Read the model definition and answer for the solid it produces. Units are mm, in the model's axes. A direction names the side the tool comes from. Give positions to 0.01 mm unless a question says otherwise; leave off trailing zeros. Order: outer loops, then holes, each group sorted by start corner. A loop starts at its lowest first (then second) coordinate and runs counter-clockwise, first axis right, second up. Notation, with made-up numbers: (-1.5, 61.25) -> (21.5, 61.25) arc R27 ccw to (21.5, 85.25) -> close; hole circle Ø11 at (6, 80). An arc over 180 degrees is marked (long way). Answer as CSV lines item,"result". Start each with the question number.
1) Find section A-A (x = 13.5). Determine the outline of the cut face in (y, z), and give its area (3 significant figures).
2) Find section C-C (y = 13). Determine the outline of the cut face in (x, z), and give its area (3 significant figures).
3) Flat-ended cylindrical pins translate along their axes: pin 1 Ø4 at (x, y) = (-1, 3) entering from +Z; pin 2 Ø3.5 at (y, z) = (-7.73, 35.28) entering from +X; pin 3 Ø4 at (y, z) = (14, 2) entering from -X; pin 4 Ø4 at (x, z) = (-11, 1.5) entering from +Y. Find the tip coordinate at first contact, or state that the pin passes through.
4) The mould has two halves that part along Z. Classify faces 1 (the face through (8.42, -20.77, 34.06)), 2 (the face through (20.77, 23.57, 21)), 3 (the face through (2, -19, 19)), 4 (the face through (20.774, 17.714, 11.718)): +Z half, -Z half, draft (parallel to the pull), parting line (faces both ways), or undercut.
5) Straight lines are drawn through the part: L1, parallel to Z at x = -6, y = -11.5; L2, parallel to Z at x = 20.5, y = 17; L3, parallel to X at y = 11, z = 18. For each, find the intervals that lie inside material, in ascending order. Write a range as from..to.
6) For faces 5 (the face through (22.5, -1, 20)), 6 (the face through (19, -2, 19)), 7 (the face through (21, 14, 22.5)), 8 (the face through (-3.5, -21, 33)), determine the directions among +Z, -Z, +X, -X, +Y, -Y from which every point of the face is accessible in a straight line to the end or side of a thin tool.
7) Find section B-B (x = -17). Determine the outline of the cut face in (y, z), and give its area (3 significant figures).
```python
from build123d import *

# Parameters (mm, degrees)
F1_DEPTH  = 44
F2_T      = -3.5
F3_W      = 21.5
F3_H      = 21.5
F4_DEPTH  = 25
F5_W      = 21.5
F5_H      = 21.5
F6_DEPTH  = 25
F7_R      = 5
F10_R     = 1.5
F11_DEPTH = 25
F9_R      = 1.5
F12_DEPTH = 25
F8_R      = 1.5
F13_DEPTH = 25


with BuildPart() as f1:
    # F0 (on Top) → F1 (new body)
    with BuildSketch(Plane.XY):
        Polygon((0, 25), (0, 0), (-25, 0), (-25, -22.5), (0, -22.5), (22.5, -22.5), (22.5, 0), (22.5, 25), align=None)
    extrude(amount=F1_DEPTH)

    # F2
    f2_openings = [f1.faces().sort_by_distance(p)[0] for p in [
        (3.060345, -3.060345, 44),
        (0, 12.5, 22),
        (-12.5, 0, 22),
        (-25, -11.25, 22),
        (11.25, 25, 22),
    ]]
    offset(amount=F2_T, openings=f2_openings)

    # F3 (on face) → F4 (cut)
    with BuildSketch(Plane(origin=(19, 0, 0), x_dir=(0, -1, 0), z_dir=(-1, 0, 0))):
        with Locations((-14.25, 33.25)):
            Rectangle(F3_W, F3_H)
    extrude(amount=-F4_DEPTH, mode=Mode.SUBTRACT)

    # F5 (on face) → F6 (cut)
    with BuildSketch(Plane(origin=(0, -19, 0), x_dir=(-1, 0, 0), z_dir=(0, 1, 0))):
        with Locations((14.25, 33.25)):
            Rectangle(F5_W, F5_H)
    extrude(amount=-F6_DEPTH, mode=Mode.SUBTRACT)

    # F7
    f7_edges = [f1.edges().sort_by_distance(p)[0] for p in [
        (22.5, 1.25, 0),
        (-1.25, -22.5, 0),
        (22.5, -22.5, 22),
        (0, 0, 1.75),
        (-3.5, -20.75, 22.5),
        (0, 25, 1.75),
        (20.75, 25, 22.5),
        (-3.5, -20.75, 44),
        (-25, -20.75, 22.5),
        (-25, 0, 1.75),
        (20.75, 3.5, 22.5),
        (20.75, 3.5, 44),
    ]]
    fillet(f7_edges, radius=F7_R)

    # F10 (on face) → F11 (cut)
    with BuildSketch(Plane.XZ.offset(22.5)):
        with Locations((7.732233047, 35.3934139763)):
            Circle(F10_R)
        with Locations((-16.3934139763, 11.267766953)):
            Circle(F10_R)
    extrude(amount=-F11_DEPTH, mode=Mode.SUBTRACT)

    # F9 (on face) → F12 (cut)
    with BuildSketch(Plane.YZ.offset(22.5)):
        with Locations((-7.732233047, 35.2836836879)):
            Circle(F9_R)
        with Locations((16.2836836879, 11.267766953)):
            Circle(F9_R)
    extrude(amount=-F12_DEPTH, mode=Mode.SUBTRACT)

    # F8 (on face) → F13 (cut)
    with BuildSketch(Plane.XY.offset(3.5)):
        with Locations((-17.0746488054, -8.482233047)):
            Circle(F8_R)
        with Locations((8.482233047, 17.0746488054)):
            Circle(F8_R)
    extrude(amount=-F13_DEPTH, mode=Mode.SUBTRACT)


solid = f1.part
```
Findings below:
1,outline,"(-22.5, 5) arc R5 ccw to (-17.5, 0) -> (25, 0) -> (25, 3.5) -> (-19, 3.5) -> (-19, 44) -> (-22.5, 44) -> close"
1,area,"303 mm²"
2,outline,"(0, 0) -> (17.5, 0) arc R5 ccw to (22.5, 5) -> (22.5, 22.5) -> (19, 22.5) -> (19, 3.5) -> (0, 3.5) -> close"
2,area,"140 mm²"
3,pin 1,"z = 3.5"
3,pin 2,"x = 22.5"
3,pin 3,"x = 0"
3,pin 4,"y = 0"
4,face 1,"undercut"
4,face 2,"+Z half"
4,face 3,"draft"
4,face 4,"undercut"
5,L1,"0..3.5"
5,L2,"1..9.95, 12.59..22.5"
5,L3,"19..22.5"
6,face 5,"+Z, -Z, +X, +Y, -Y"
6,face 6,"+Z, -X, +Y"
6,face 7,"+Z, +X, -X, +Y"
6,face 8,"+Z, -X, +Y, -Y"
7,outline,"(-22.5, 5) arc R5 ccw to (-17.5, 0) -> (-9.98, 0) -> (-9.98, 3.5) -> (-19, 3.5) -> (-19, 9.9) -> (-22.5, 9.9) -> close; (-22.5, 12.64) -> (-19, 12.64) -> (-19, 22.5) -> (-22.5, 22.5) -> close; (-6.98, 0) -> (0, 0) -> (0, 3.5) -> (-6.98, 3.5) -> close"
7,area,"120 mm²"
